The listing builds one solid part. Answer for the finished solid, in the listing's coordinates (mm). A direction names the side the tool comes from. Give positions to 0.01 mm unless a question says otherwise; leave off trailing zeros. Order: outer loops, then holes, each group sorted by start corner. A loop starts at its lowest first (then second) coordinate and runs counter-clockwise, first axis right, second up. Notation, with made-up numbers: (55, -22) - (69, -22) arc R17 ccw to (69, -18) - close; hole circle Ø3 at (12, -22.5). An arc over 180 degrees is marked (long way). Answer as CSV lines item,"result". Start each with the question number.
1. Which of the six approach directions +Z, -Z, +X, -X, +Y, -Y give full straight-line access (tool end or side, diameter ignored) to faces 4 (the cylindrical face through (236.12, 2.96, 4.09)), 5 (the cylindrical face through (256.35, 2.96, 222.14)), 6 (the cylindrical face through (236.09, 2.96, -14.45))?
2. Flat-ended cylindrical pins translate along their axes: pin 1 (3 mm diameter, centred on x = 125, y = 5, fed in from +Z); pin 2 (1.8 mm diameter, centred on x = -46, y = 4.5, fed in from -Z); pin 3 (1.5 mm diameter, centred on y = 2, z = -9.5, fed in from -X). Find the tip coordinate at first contact, or state that the pin passes through.
3. Consider line 1 along Z through (x, y) = (200, 1.9); line 2 along X through (y, z) = (4.4, 109); line 3 along X through (y, z) = (0.85, -34.5). Determine where each line is inside the solid, lowest interval first. Write a range as [from, to].
4. Determine the mould class of faces 1 (the cylindrical face through (-236.34, 2.96, 4.31)), 2 (the cylindrical face through (-235.864, 2.958, -14.235)), 3 (the cylindrical face through (-255.718, 2.958, 222.133)) for opening direction Z: +Z half, -Z half, draft (parallel to the pull), parting line (faces both ways), or undercut.
5. Section A-A on x = -143 is taken. Give the vertices of the cut face in (y, z), and give its area (3 significant figures).
6. Section B-B on z = -75.5 is taken. Give the vertices of the cut face in (x, y), and give its area (3 significant figures).
7. Section D-D on x = 256.15 is taken. Give the vertices of the cut face in (y, z).
Solid Edge part; units mm, degrees
sketch "Sketch1" plane through (0, 0, 0) normal (0, -1, 0) x (1, 0, 0)
  line L0 (241.81, 14.34) -> (241.81, 207.8)
  arc A0 (241.81, 207.8) -> (270.488, 208.0371) centre (256.15, 207.8) cw
  line L1 (270.488, 208.0371) -> (276.8881, -178.9518)
  arc A1 (276.8881, -178.9518) -> (249.5268, -179.8566) centre (263.2, -179.1781) cw
  line L2 (241.7907, -23.9491) -> (249.5268, -179.8566)
  arc A2 (241.7907, -23.9491) -> (226.09, -9.0081) centre (226.09, -24.7281) ccw
  line L3 (226.09, -9.0081) -> (0, -9.0081)
  line L4 (-226.09, -9.0081) -> (0, -9.0081)
  arc A3 (-241.7907, -23.9491) -> (-226.09, -9.0081) centre (-226.09, -24.7281) cw
  line L5 (-241.7907, -23.9491) -> (-249.5268, -179.8566)
  arc A4 (-276.8881, -178.9518) -> (-249.5268, -179.8566) centre (-263.2, -179.1781) ccw
  line L6 (-270.488, 208.0371) -> (-276.8881, -178.9518)
  arc A5 (-241.81, 207.8) -> (-270.488, 208.0371) centre (-256.15, 207.8) ccw
  line L7 (-241.81, 14.34) -> (-241.81, 207.8)
  arc A6 (-226.09, -1.38) -> (-241.81, 14.34) centre (-226.09, 14.34) cw
  line L8 (0, -1.38) -> (-226.09, -1.38)
  line L9 (0, -1.38) -> (226.09, -1.38)
  arc A7 (226.09, -1.38) -> (241.81, 14.34) centre (226.09, 14.34) ccw
  line L10 (240.43, 14.34) -> (240.43, 207.8)
  arc A8 (240.43, 207.8) -> (271.868, 208.0599) centre (256.1501, 207.8) cw
  line L11 (271.868, 208.0599) -> (278.2681, -178.9289)
  arc A9 (248.1483, -179.925) -> (278.2681, -178.9289) centre (263.2, -179.1781) ccw
  line L12 (240.4124, -24.0175) -> (248.1483, -179.925)
  arc A10 (226.09, -10.3881) -> (240.4124, -24.0175) centre (226.09, -24.7281) cw
  line L13 (0, -10.3881) -> (226.09, -10.3881)
  line L14 (0, -10.3881) -> (-226.09, -10.3881)
  arc A11 (-226.09, -10.3881) -> (-240.4124, -24.0175) centre (-226.09, -24.7281) ccw
  line L15 (-240.4124, -24.0175) -> (-248.1483, -179.925)
  arc A12 (-248.1483, -179.925) -> (-278.2681, -178.9289) centre (-263.2, -179.1781) cw
  line L16 (-271.868, 208.0599) -> (-278.2681, -178.9289)
  arc A13 (-240.43, 207.8) -> (-271.868, 208.0599) centre (-256.1501, 207.8) ccw
  line L17 (-240.43, 14.34) -> (-240.43, 207.8)
  arc A14 (-226.09, 0) -> (-240.43, 14.34) centre (-226.09, 14.34) cw
  line L18 (0, 0) -> (-226.09, 0)
  line L19 (0, 0) -> (226.09, 0)
  arc A15 (226.09, 0) -> (240.43, 14.34) centre (226.09, 14.34) ccw
extrude "Protrusion1" add sketch "Sketch1" against normal blind 6
Checks:
1,face 4,"+Z, +Y, -Y"
1,face 5,"+Y, -Y"
1,face 6,"-Z, +Y, -Y"
2,pin 1,"stops at z = 0"
2,pin 2,"stops at z = -10.39"
2,pin 3,"stops at x = -275.48"
3,line 1,"z = [-10.39, -9.01], [-1.38, 0]"
3,line 2,"x = [-273.51, -272.13], [-241.81, -240.43], [240.43, 241.81], [272.13, 273.51]"
3,line 3,"x = [-275.88, -274.5], [-242.31, -240.93], [240.93, 242.31], [274.5, 275.88]"
4,face 1,"+Z half"
4,face 2,"-Z half"
4,face 3,"undercut"
5,outline,"(0, -10.39) - (6, -10.39) - (6, -9.01) - (0, -9.01) - close; (0, -1.38) - (6, -1.38) - (6, 0) - (0, 0) - close"
5,area,"16.6 mm²"
6,outline,"(-276.56, 0) - (-275.18, 0) - (-275.18, 6) - (-276.56, 6) - close; (-244.35, 0) - (-242.97, 0) - (-242.97, 6) - (-244.35, 6) - close; (242.97, 0) - (244.35, 0) - (244.35, 6) - (242.97, 6) - close; (275.18, 0) - (276.56, 0) - (276.56, 6) - (275.18, 6) - close"
6,area,"33.1 mm²"
7,outline,"(0, -192.5) - (6, -192.5) - (6, -190.91) - (0, -190.91) - close; (0, 222.14) - (6, 222.14) - (6, 223.52) - (0, 223.52) - close"
